Model file for the job. Use its own axes, mm. Coordinates: 2 decimals unless noted, no trailing zeros. Order: outer loops, then holes, each group sorted by start corner. A loop starts at its lowest first (then second) coordinate and runs counter-clockwise, first axis right, second up. Notation, with made-up numbers: (37, 44.5) -> (64, 44.5) arc R10 ccw to (64, 56.5) -> close; hole circle Ø1 at (36.5, 11.25). An arc over 180 degrees is marked (long way). Return JSON: item names as keys, results as strings. Group by question number.
1) Probe line 1 (Z direction, x = 21, y = 190); line 2 (Z direction, x = 1, y = 88.5); line 3 (X direction, y = 221, z = 10). List the from-to ranges inside material, lowest first.
2) Cut at A-A (y = 139.7). Write the cut outline in (x, z), and give its area (3 significant figures).
3) Cut at B-B (x = 3). State how many separate pieces and enclosed holes the cut face has, and give its area (3 significant figures).
4) Flat gauge pins, fed straight in: pin 1 (11.5 mm diameter, centred on y = 168, z = 11.5, fed in from +X); pin 2 (6 mm diameter, centred on y = 88.9, z = -12.7, fed in from -X); pin 3 (7 mm diameter, centred on y = 39, z = -15.5, fed in from +X). Where does each tip first touch, or does it go through?
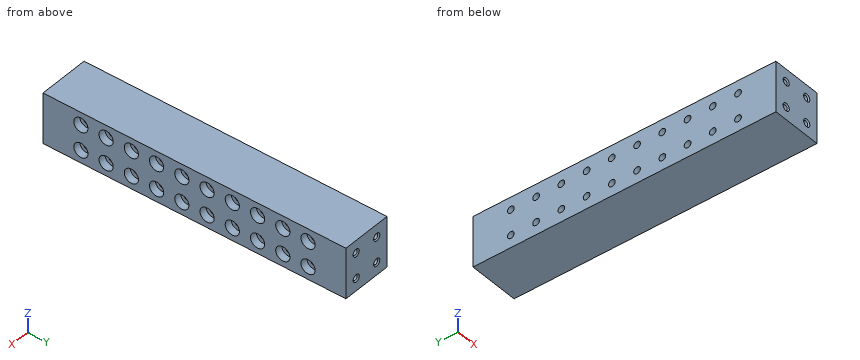
from build123d import *

# Parameters (mm, degrees)
SKETCH1_W                                            = 50.8
SKETCH1_H                                            = 50.8
BOSS_EXTRUDE1_DEPTH                                  = 304.8
F_1_4_20_TAPPED_HOLE1_AT_2_COUNT                     = 2
F_1_4_20_TAPPED_HOLE1_AT_2_PITCH                     = 25.4
F_1_4_20_TAPPED_HOLE1_AT_3_COUNT                     = 2
F_1_4_20_TAPPED_HOLE1_AT_3_PITCH                     = 35.921024484
F_1_4_20_TAPPED_HOLE1_AT_4_COUNT                     = 2
F_1_4_20_TAPPED_HOLE1_AT_4_PITCH                     = 25.4
CBORE_FOR_1_4_BINDING_HEAD_MACHINE_SCREW_D           = 6.7564
CBORE_FOR_1_4_BINDING_HEAD_MACHINE_SCREW_CBORE_D     = 14.2875
CBORE_FOR_1_4_BINDING_HEAD_MACHINE_SCREW_CBORE_DEPTH = 7.366


with BuildPart() as part:
    # Sketch1 → Boss-Extrude1 (new body)
    with BuildSketch(Plane(origin=(0, 0, 0), x_dir=(1, 0, 0), z_dir=(0, 1, 0))):
        Rectangle(SKETCH1_W, SKETCH1_H)
    extrude(amount=BOSS_EXTRUDE1_DEPTH)

    # Sketch3 → 1/4-20 Tapped Hole1 (revolve, cut)
    with BuildSketch(Plane(origin=(-12.7, 304.8, -12.7), x_dir=(0, 0, 1), z_dir=(1, 0, 0))):
        Polygon((0, 0), (0, 26.933816902), (2.5527, 25.4), (2.5527, 1.054999966), (3.81, 0), align=None)
    f_1_4_20_tapped_hole1 = revolve(axis=Axis((-12.7, 311.15, -12.7), (0, -1, 0)), mode=Mode.SUBTRACT)

    # 1/4-20 Tapped Hole1 at 2: 1/4-20 Tapped Hole1 ×2
    with Locations(*[(i * F_1_4_20_TAPPED_HOLE1_AT_2_PITCH, 0, 0) for i in range(1, F_1_4_20_TAPPED_HOLE1_AT_2_COUNT)]):
        add(f_1_4_20_tapped_hole1, mode=Mode.SUBTRACT)

    # 1/4-20 Tapped Hole1 at 3: 1/4-20 Tapped Hole1 ×2
    with Locations(*[Vector(0.7071067811865476, 0, 0.7071067811865475) * (i * F_1_4_20_TAPPED_HOLE1_AT_3_PITCH) for i in range(1, F_1_4_20_TAPPED_HOLE1_AT_3_COUNT)]):
        add(f_1_4_20_tapped_hole1, mode=Mode.SUBTRACT)

    # 1/4-20 Tapped Hole1 at 4: 1/4-20 Tapped Hole1 ×2
    with Locations(*[(0, 0, i * F_1_4_20_TAPPED_HOLE1_AT_4_PITCH) for i in range(1, F_1_4_20_TAPPED_HOLE1_AT_4_COUNT)]):
        add(f_1_4_20_tapped_hole1, mode=Mode.SUBTRACT)

    # Mirror1: 1/4-20 Tapped Hole1 across plane
    add(f_1_4_20_tapped_hole1.mirror(Plane(origin=(0, 152.4, 0), x_dir=(0, 0, 1), z_dir=(0, -1, 0))), mode=Mode.SUBTRACT)

    # Mirror1 copy 1 sketch → Mirror1 copy 1 (revolve, cut)
    with BuildSketch(Plane(origin=(12.7, 0, -12.7), x_dir=(0, 0, 1), z_dir=(1, 0, 0))):
        Polygon((0, 0), (0, -26.933816902), (2.5527, -25.4), (2.5527, -1.054999966), (3.81, 0), align=None)
    revolve(axis=Axis((12.7, -6.35, -12.7), (0, -1, 0)), mode=Mode.SUBTRACT)

    # Mirror1 copy 2 sketch → Mirror1 copy 2 (revolve, cut)
    with BuildSketch(Plane(origin=(12.7, 0, 12.7), x_dir=(0, 0, 1), z_dir=(1, 0, 0))):
        Polygon((0, 0), (0, -26.933816902), (2.5527, -25.4), (2.5527, -1.054999966), (3.81, 0), align=None)
    revolve(axis=Axis((12.7, -6.35, 12.7), (0, -1, 0)), mode=Mode.SUBTRACT)

    # Mirror1 copy 3 sketch → Mirror1 copy 3 (revolve, cut)
    with BuildSketch(Plane(origin=(-12.7, 0, 12.7), x_dir=(0, 0, 1), z_dir=(1, 0, 0))):
        Polygon((0, 0), (0, -26.933816902), (2.5527, -25.4), (2.5527, -1.054999966), (3.81, 0), align=None)
    revolve(axis=Axis((-12.7, -6.35, 12.7), (0, -1, 0)), mode=Mode.SUBTRACT)

    # CBORE for 1/4 Binding Head Machine Screw1 (through all)
    with Locations(Plane(origin=(25.4, 0, 0), x_dir=(0, 0, -1), z_dir=(1, 0, 0))):
        with Locations((-12.7, 266.7), (12.7, 266.7), (12.7, 241.3), (12.7, 215.9), (12.7, 190.5), (-12.7, 241.3), (-12.7, 215.9), (-12.7, 190.5), (-12.7, 165.1), (12.7, 165.1), (-12.7, 139.7), (12.7, 139.7), (-12.7, 114.3), (12.7, 114.3), (-12.7, 88.9), (12.7, 88.9), (-12.7, 63.5), (12.7, 63.5), (-12.7, 38.1), (12.7, 38.1)):
            CounterBoreHole(CBORE_FOR_1_4_BINDING_HEAD_MACHINE_SCREW_D / 2, CBORE_FOR_1_4_BINDING_HEAD_MACHINE_SCREW_CBORE_D / 2, CBORE_FOR_1_4_BINDING_HEAD_MACHINE_SCREW_CBORE_DEPTH)


solid = part.part
Answers below:
{
 "1": {"line 1": "z = -25.4 to -19.83, -5.57 to 5.57, 19.83 to 25.4", "line 2": "z = -25.4 to -16.05, -9.35 to 9.35, 16.05 to 25.4", "line 3": "x = -25.4 to 18.03"},
 "2": {"outline": "(-25.4, -25.4) -> (25.4, -25.4) -> (25.4, -19.84) -> (18.03, -19.84) -> (18.03, -16.08) -> (-25.4, -16.08) -> close; (-25.4, -9.32) -> (18.03, -9.32) -> (18.03, -5.56) -> (25.4, -5.56) -> (25.4, 5.56) -> (18.03, 5.56) -> (18.03, 9.32) -> (-25.4, 9.32) -> close; (-25.4, 16.08) -> (18.03, 16.08) -> (18.03, 19.84) -> (25.4, 19.84) -> (25.4, 25.4) -> (-25.4, 25.4) -> close", "area": "1,780 mm^2"},
 "3": {"separate pieces": "1", "enclosed holes": "20", "area": "14,800 mm^2"},
 "4": {"pin 1": "stops at x = 25.4", "pin 2": "passes through", "pin 3": "stops at x = 18.03"}
}
